from build123d import *

# Parameters (mm, degrees)
SKETCH5_W          = 8
SKETCH5_H          = 7
CUT_EXTRUDE5_DEPTH = 172.877863613
SKETCH12_R         = 6
CUT_EXTRUDE6_DEPTH = 161.832210704


with BuildPart() as part:
    # Sketch2 → Revolve3 (revolve)
    with BuildSketch(Plane(origin=(0, 0, 0), x_dir=(1, 0, 0), z_dir=(0, 1, 0)), mode=Mode.PRIVATE) as revolve3_sk:
        with BuildLine():
            Line((0, 15), (0, 111))
            Line((0, 111), (-45, 111))
            Line((-45, 111), (-45, 96))
            Line((-45, 96), (-40, 96))
            ThreePointArc((-40, 96), (-36.464466094, 94.535533906), (-35, 91))
            Line((-35, 91), (-35, 35))
            ThreePointArc((-35, 35), (-36.464466094, 31.464466094), (-40, 30))
            Line((-40, 30), (-70, 30))
            Line((-70, 30), (-70, 15))
            Line((-70, 15), (0, 15))
        make_face()
    revolve(revolve3_sk.sketch.rotate(Axis((0, 0, 0), (1, 0, 0)), 180), axis=Axis((0, 0, 0), (1, 0, 0)))

    # Sketch5 → Cut-Extrude5 (cut, through all)
    with BuildSketch(Plane.ZY.offset(70)):
        with Locations((0, 15)):
            Rectangle(SKETCH5_W, SKETCH5_H)
    extrude(amount=-CUT_EXTRUDE5_DEPTH, mode=Mode.SUBTRACT)

    # Sketch12 → Cut-Extrude6 (cut, through all)
    with BuildSketch(Plane.ZY.offset(35)):
        with Locations((51.961524227, 30)):
            Circle(SKETCH12_R)
        with Locations(Location((-51.961524227, 30, 0), (0, 0, 180))):
            Circle(SKETCH12_R)
        with Locations(Location((51.961524227, -30, 0), (0, 0, 180))):
            Circle(SKETCH12_R)
        with Locations((-51.961524227, -30)):
            Circle(SKETCH12_R)
        with Locations((0, 60)):
            Circle(SKETCH12_R)
        with Locations(Location((0, -60, 0), (0, 0, 180))):
            Circle(SKETCH12_R)
    extrude(amount=-CUT_EXTRUDE6_DEPTH, mode=Mode.SUBTRACT)


solid = part.part
Design review of the part built by this model. Coordinates are the model's own, in mm. A direction names the side the tool comes from. Round coordinates to 2 decimals unless told otherwise and drop trailing zeros. Write each loop counter-clockwise with the first axis right and the second up, starting at its lowest first coordinate (ties: lowest second). Pieces come first, ordered by that corner, then holes. Notation, with made-up numbers: (-10, -20) - (28, -20) arc R28 cw to (28, 9) - close; hole circle Ø10 at (-31, 6). An arc over 180 degrees is marked (long way). Return JSON: item names as keys, results as strings. Group by question number.
Item 1: Machinability: for faces 4 (the face through (0, 23, 2)), 5 (the face through (-35, 18.5, 0)), 6 (the face through (-42.465, -28.836, 91.567)), which of the approach directions +Z, -Z, +X, -X, +Y, -Y give a long, thin tool a straight path to every point of the face, cutting with its end or side? Answer none if there is none.
Item 2: We need section C-C on z = 51. Give the number of separate pieces and of enclosed holes in the cut face, and give its area (3 significant figures).
Item 3: We need section B-B on y = 0. Write out the cut boundary in (x, z), and give its area (3 significant figures).
Item 4: We need section A-A on z = 0. Write out the cut boundary in (x, y), and give its area (3 significant figures).
Item 5: For probe 1 along Y at (x, z) = (-10, 0); probe 2 along Y at (x, z) = (-41.2, 0); probe 3 along Z at (x, y) = (-19, -29), list the stretches that pass through material, from the lowest coordinate up. Write a range as [from, to].
Item 6: Insertion check: P1, Ø2, axis at x = -47.5, y = -85.5, coming from the +Z side; P2, Ø4.5, axis at x = -43.5, y = 17, coming from the -Z side; P3, Ø3, axis at x = -32, y = 29, coming from the +Z side; P4, Ø15.5, axis at y = -30, z = -51.96, coming from the +X side. Each pin has a flat end and moves straight along its axis. Give the tip position at first contact, or say it passes through.
Item 7: The part is to be moulded in two halves that separate along Z. For faces 1 (the face through (-22.815, -33.341, 105.874)), 2 (the face through (-70, -14, 6)), 3 (the face through (-17.745, 35.857, -50.661)), say which applies: pulls with the +Z half, pulls with the -Z half, needs draft (parallel to the pull), parting line crosses it, or undercut.
Model answer:
{
 "1": {"face 4": "+Z, -Z, +X, +Y, -Y", "face 5": "+X, -X", "face 6": "-X"},
 "2": {"separate pieces": "3", "enclosed holes": "0", "area": "6,430 mm²"},
 "3": {"outline": "(-70, -30) - (-40, -30) arc R5 cw to (-35, -35) - (-35, -91) arc R5 cw to (-40, -96) - (-45, -96) - (-45, -111) - (0, -111) - (0, -15) - (-70, -15) - close; (-70, 15) - (0, 15) - (0, 111) - (-45, 111) - (-45, 96) - (-40, 96) arc R5 cw to (-35, 91) - (-35, 35) arc R5 cw to (-40, 30) - (-70, 30) - close", "area": "8,090 mm²"},
 "4": {"outline": "(-70, -30) - (-40, -30) arc R5 cw to (-35, -35) - (-35, -54) - (0, -54) - (0, -15) - (-70, -15) - close; (-70, 18.5) - (0, 18.5) - (0, 54) - (-35, 54) - (-35, 35) arc R5 cw to (-40, 30) - (-70, 30) - close; (-45, -111) - (0, -111) - (0, -66) - (-35, -66) - (-35, -91) arc R5 cw to (-40, -96) - (-45, -96) - close; (-45, 96) - (-40, 96) arc R5 cw to (-35, 91) - (-35, 66) - (0, 66) - (0, 111) - (-45, 111) - close", "area": "7,010 mm²"},
 "5": {"probe 1": "y = [-111, -66], [-54, -15], [18.5, 54], [66, 111]", "probe 2": "y = [-111, -96], [-30, -15], [18.5, 30], [96, 111]", "probe 3": "z = [-107.14, -57.88], [-46.05, 46.05], [57.88, 107.14]"},
 "6": {"P1": "passes through", "P2": "stops at z = -110.02", "P3": "stops at z = 107.54", "P4": "stops at x = 0"},
 "7": {"face 1": "parting line crosses it", "face 2": "needs draft", "face 3": "undercut"}
}
